Build history of the part. All positions in model axes, mm. Face numbers are marked on the shaded views. A direction names the side the tool comes from. Give positions to 0.01 mm unless a question says otherwise; leave off trailing zeros. Write each loop counter-clockwise with the first axis right and the second up, starting at its lowest first coordinate (ties: lowest second). Pieces come first, ordered by that corner, then holes. Notation, with made-up numbers: (75, -20.75) -> (96, -20.75) arc R34 ccw to (96, 11.25) -> close; hole circle Ø4 at (-14.5, 77.5). An arc over 180 degrees is marked (long way). One line per question, with ' | ' between items. Start each with the question number.
(1) Band-saw the part on C-C, the plane x = 43. Give the cut face in (y, z).
(2) Pin check, flat tip, straight feed: P1, Ø16, axis at x = 20.5, y = 9, coming from the +Z side. Stop position of the tip, or through.
(3) Band-saw the part on A-A, the plane y = 4.5. Give the cut face in (x, z), and give its area (3 significant figures).
(4) Band-saw the part on B-B, the plane z = 5.25. Give the cut face in (x, y), and give its area (3 significant figures).
(5) Pull direction X, two halves, no side cores. Call the marked faces 3, 4 and 5: released by +X, released by -X, zero draft, split by the parting line, or undercut.
(6) Drill centre lines: probe 1 along Y at (x, z) = (32.5, 7.5); probe 2 along X at (y, z) = (21.5, 3); probe 3 along Z at (x, y) = (39.5, 7). Where is each one in solid material? Low to high. Write a range as from..to.
(7) Tool access for the marked faces 1 and 2: list every direction of +Z, -Z, +X, -X, +Y, -Y with a clear straight run to the whole face (end or side of a thin tool).
Autodesk Fusion 360 part; units mm, degrees
sketch "Sketch1" plane through (0, 0, 0) normal (0, 0, 1) x (1, 0, 0)
  line L0 (0, 0) -> (46, 0)
  line L1 (46, 0) -> (46, 32)
  line L2 (46, 32) -> (0, 32)
  line L3 (0, 32) -> (0, 0)
  line L4 (-2, 34) -> (48, 34)
  line L5 (48, 34) -> (48, -2)
  line L6 (48, -2) -> (-2, -2)
  line L7 (-2, -2) -> (-2, 34)
  dimension "d1" = 46
  dimension "d2" = 32
  dimension "d3" = 2
  dimension "d4" = 2
  dimension "d5" = 2
  dimension "d6" = 2
extrude "Extrude1" add sketch "Sketch1" along normal blind 2 contours L0 L1 L2 L3
extrude "Extrude2" add sketch "Sketch1" along normal blind 10
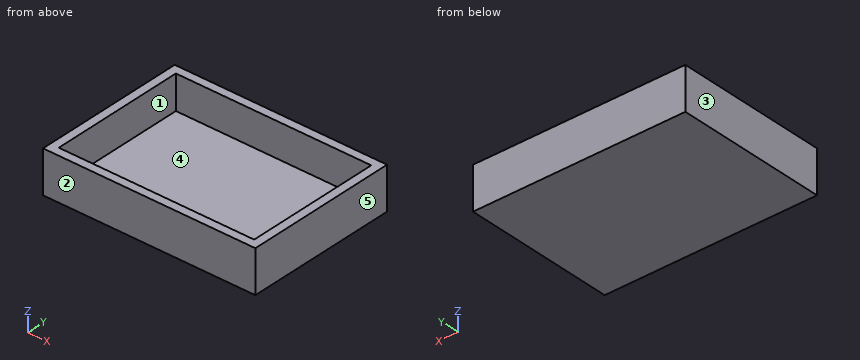
Results:
1) outline: (-2, 0) -> (34, 0) -> (34, 10) -> (32, 10) -> (32, 2) -> (0, 2) -> (0, 10) -> (-2, 10) -> close
2) P1: stops at z = 2
3) outline: (-2, 0) -> (48, 0) -> (48, 10) -> (46, 10) -> (46, 2) -> (0, 2) -> (0, 10) -> (-2, 10) -> close | area: 132 mm²
4) outline: (-2, -2) -> (48, -2) -> (48, 34) -> (-2, 34) -> close; hole (0, 0) -> (46, 0) -> (46, 32) -> (0, 32) -> close | area: 328 mm²
5) face 3: released by -X | face 4: undercut | face 5: released by +X
6) probe 1: y = -2..0, 32..34 | probe 2: x = -2..0, 46..48 | probe 3: z = 0..2
7) face 1: +Z | face 2: +Z, -Z, +X, -X, -Y
